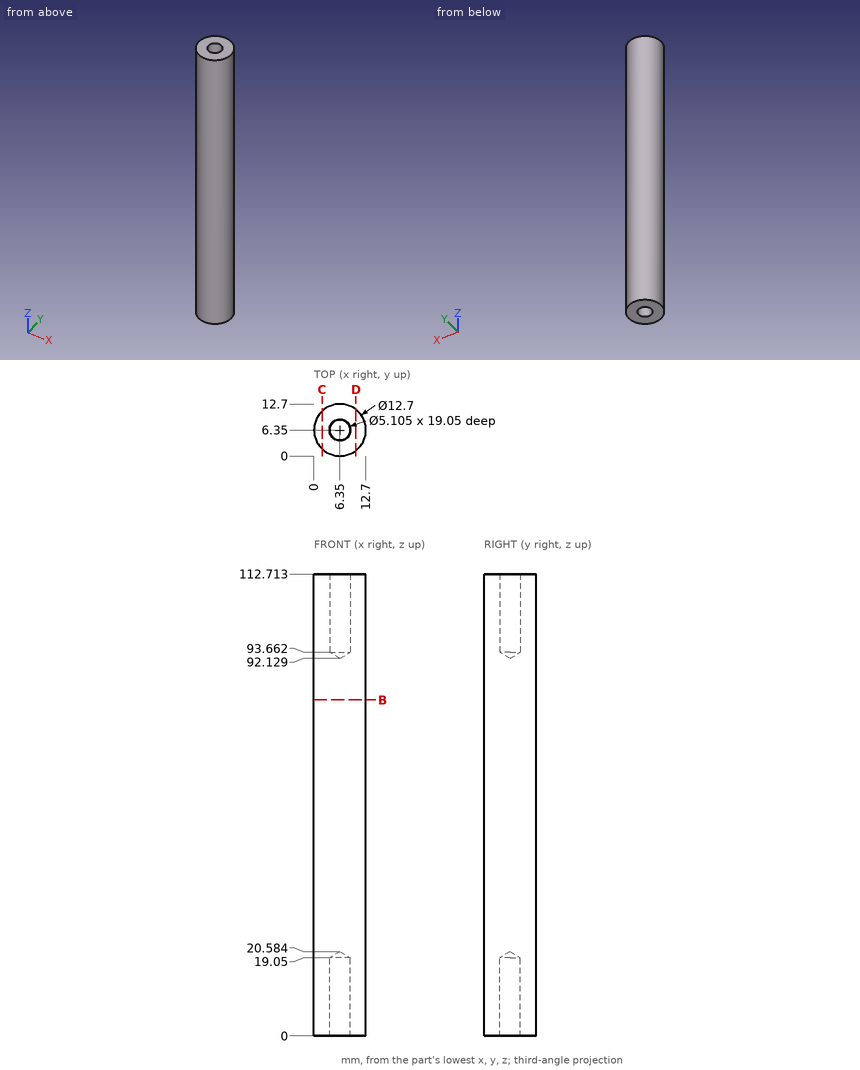
Check sheet for the drawn part. Datum: minimum x, y, z corner. Units: mm. Round coordinates to 2 decimals unless told otherwise and drop trailing zeros. Order: outer loops, then holes, each group sorted by start corner. A loop starts at its lowest first (then second) coordinate and runs counter-clockwise, first axis right, second up.
1) Section check D-D (x = 10.25). Record the boundary of the cut face in (y, z).
2) Section check B-B (z = 82). Record the boundary of the cut face in (x, y).
3) Scan lines: line 1 (Y direction, x = 6.35, z = 7.5); line 2 (X direction, y = 6, z = 64.5); line 3 (Y direction, x = 6.5, z = 85.5). Record each from-to range of solid material in increasing order.
4) Go/stop test with flat-tipped pins: pin 1 Ø1 at (x, z) = (5.5, 68.5) entering from -Y; pin 2 Ø4 at (x, y) = (6.35, 6.35) entering from +Z; pin 3 Ø4 at (x, z) = (2, 59) entering from +Y. Record where each tip stops, or that it passes through.
5) Section check C-C (x = 2). Record the boundary of the cut face in (y, z), and give its area (3 significant figures).
Result:
1. outline: (1.34, 0) - (11.36, 0) - (11.36, 112.71) - (1.34, 112.71) - close
2. outline: circle Ø12.7 at (6.35, 6.35)
3. line 1: y = 0 to 3.8, 8.9 to 12.7
3. line 2: x = 0.01 to 12.69
3. line 3: y = 0 to 12.7
4. pin 1: stops at y = 0.01
4. pin 2: stops at z = 93.33
4. pin 3: stops at y = 12.25
5. outline: (1.72, 0) - (10.98, 0) - (10.98, 112.71) - (1.72, 112.71) - close
5. area: 1,040 mm2
